The listing builds one solid part. Answer for the finished solid, in the listing's coordinates (mm). Face numbers are marked on the shaded views. A direction names the side the tool comes from. Coordinates: 2 decimals unless noted, no trailing zeros. Loops run counter-clockwise (first coordinate to the right, second up) from the corner with the lowest first, then second, coordinate; pieces in that order, holes last. Notation, with made-up numbers: (-22.5, 31.5) - (-7.5, 31.5) arc R15 ccw to (-7.5, 44.5) - close; hole circle Ø3 at (44.25, 19). An arc over 180 degrees is marked (long way). Use one line per item in the form item = value. Start each with the question number.
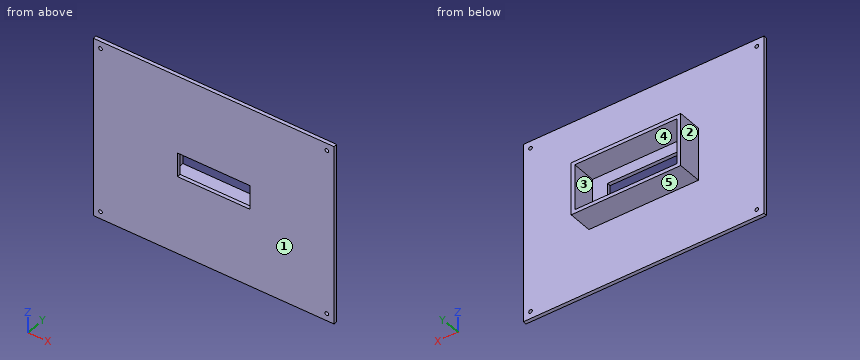
```python
from build123d import *

# Parameters (mm, degrees)
SKETCH1_W           = 200
SKETCH1_H           = 150
BOSS_EXTRUDE1_DEPTH = 3
SKETCH2_R           = 1.5
CUT_EXTRUDE1_DEPTH  = 126.035994817
SKETCH3_W           = 60
SKETCH3_H           = 20
CUT_EXTRUDE2_DEPTH  = 126.035994817
SKETCH4_W           = 91
SKETCH4_H           = 44
SKETCH4_W_2         = 85
SKETCH4_H_2         = 38
BOSS_EXTRUDE2_DEPTH = 20


with BuildPart() as part:
    # Sketch1 → Boss-Extrude1 (new body)
    with BuildSketch(Plane(origin=(0, 0, 0), x_dir=(1, 0, 0), z_dir=(0, 1, 0))):
        Rectangle(SKETCH1_W, SKETCH1_H)
    extrude(amount=BOSS_EXTRUDE1_DEPTH)

    # Sketch2 → Cut-Extrude1 (cut, through all)
    with BuildSketch(Plane(origin=(0, 3, 0), x_dir=(1, 0, 0), z_dir=(0, 1, 0))):
        with Locations(Location((94, -69, 0), (0, 0, 270))):
            Circle(SKETCH2_R)
        with Locations(Location((94, 69, 0), (0, 0, 90))):
            Circle(SKETCH2_R)
        with Locations(Location((-94, -69, 0), (0, 0, 90))):
            Circle(SKETCH2_R)
        with Locations(Location((-94, 69, 0), (0, 0, 270))):
            Circle(SKETCH2_R)
    extrude(amount=-CUT_EXTRUDE1_DEPTH, mode=Mode.SUBTRACT)

    # Sketch3 → Cut-Extrude2 (cut, through all)
    with BuildSketch(Plane(origin=(0, 3, 0), x_dir=(1, 0, 0), z_dir=(0, 1, 0))):
        Rectangle(SKETCH3_W, SKETCH3_H)
    extrude(amount=-CUT_EXTRUDE2_DEPTH, mode=Mode.SUBTRACT)

    # Sketch4 → Boss-Extrude2 (add)
    with BuildSketch(Plane(origin=(0, 3, 0), x_dir=(1, 0, 0), z_dir=(0, 1, 0))):
        Rectangle(SKETCH4_W, SKETCH4_H)
        Rectangle(SKETCH4_W_2, SKETCH4_H_2, mode=Mode.SUBTRACT)
    extrude(amount=BOSS_EXTRUDE2_DEPTH)


solid = part.part
```
(1) Determine the mould class of the marked faces 1, 2 and 3 for opening direction X: +X half, -X half, draft (parallel to the pull), parting line (faces both ways), or undercut.
(2) Find the intervals of material crossed by probe 1 along X at (y, z) = (1.6, 69); probe 2 along Z at (x, y) = (-94, 1.7); probe 3 along Z at (x, y) = (-2, 7.75), in increasing order. Write a range as from..to.
(3) A cutting plane is placed at C-C (y = 19.25). Determine the outline of the cut face in (x, z).
(4) Each of these flat-tipped pins is pushed along its axis until it touches: pin 1 Ø10 at (x, y) = (-2, 14) entering from -Z; pin 2 Ø19 at (x, z) = (-12, 5.5) entering from +Y; pin 3 Ø1.5 at (y, z) = (4, -6) entering from +X; pin 4 Ø2.5 at (x, z) = (94, -69) entering from -Y. Where does it stop, or does it pass through?
(5) For the marked faces 4 and 5, determine the directions among +Z, -Z, +X, -X, +Y, -Y from which every point of the face is accessible in a straight line to the end or side of a thin tool.
(6) A cutting plane is placed at D-D (z = -16.5). Determine the outline of the cut face in (x, y).
(7) A cutting plane is placed at B-B (x = 1). Determine the outline of the cut face in (y, z).
(8) A cutting plane is placed at A-A (z = 3). Determine the outline of the cut face in (x, y).
Evaluation:
q1.face_1 = draft
q1.face_2 = -X half
q1.face_3 = undercut
q2.probe_1 = -100..-95.5, -92.5..92.5, 95.5..100
q2.probe_2 = -75..-70.5, -67.5..67.5, 70.5..75
q2.probe_3 = -22..-19, 19..22
q3.outline = (-45.5, -22) - (45.5, -22) - (45.5, 22) - (-45.5, 22) - close; hole (-42.5, -19) - (42.5, -19) - (42.5, 19) - (-42.5, 19) - close
q4.pin_1 = -22
q4.pin_2 = 3
q4.pin_3 = 45.5
q4.pin_4 = through
q5.face_4 = +Y
q5.face_5 = -Z, +X, -X, +Y
q6.outline = (-100, 0) - (100, 0) - (100, 3) - (45.5, 3) - (45.5, 23) - (42.5, 23) - (42.5, 3) - (-42.5, 3) - (-42.5, 23) - (-45.5, 23) - (-45.5, 3) - (-100, 3) - close
q7.outline = (0, -75) - (3, -75) - (3, -22) - (23, -22) - (23, -19) - (3, -19) - (3, -10) - (0, -10) - close; (0, 10) - (3, 10) - (3, 19) - (23, 19) - (23, 22) - (3, 22) - (3, 75) - (0, 75) - close
q8.outline = (-100, 0) - (-30, 0) - (-30, 3) - (-42.5, 3) - (-42.5, 23) - (-45.5, 23) - (-45.5, 3) - (-100, 3) - close; (30, 0) - (100, 0) - (100, 3) - (45.5, 3) - (45.5, 23) - (42.5, 23) - (42.5, 3) - (30, 3) - close
